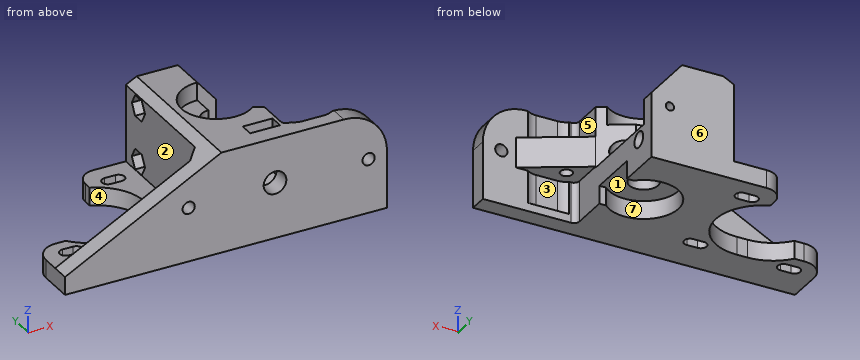
```python
from build123d import *

# Parameters (mm, degrees)
SKETCH1_R                = 4
BOSS_EXTRUDE1_DEPTH      = 28
SKETCH2_W                = 40.5
SKETCH2_H                = 38
CUT_EXTRUDE1_DEPTH       = 23
SKETCH3_R                = 9.65
CUT_EXTRUDE2_DEPTH       = 5
SKETCH8_R                = 1.15
CUT_EXTRUDE7_DEPTH       = 44
CHAMFER1_SIZE            = 23
CHAMFER1_SIZE2           = 43.5
SKETCH9_R                = 2.2
CUT_EXTRUDE8_DEPTH       = 90.5
CUT_EXTRUDE9_DEPTH       = 3
CUT_EXTRUDE9_DEPTH_BACK  = 4
CHAMFER2_SIZE            = 3
SKETCH16_W               = 26
SKETCH16_H               = 38
CUT_EXTRUDE12_DEPTH      = 29.0000001
CUT_EXTRUDE3_DEPTH       = 5
FILLET6_R                = 1.5
CUT_EXTRUDE13_DEPTH      = 17
SKETCH21_R               = 1.65
BOSS_EXTRUDE3_DEPTH      = 4.2
BOSS_EXTRUDE3_DEPTH_BACK = 4.2
SKETCH15_R               = 1.7
CUT_EXTRUDE11_DEPTH      = 44
CUT_EXTRUDE14_DEPTH      = 9
CHAMFER4_SIZE            = 8.5
CHAMFER4_SIZE2           = 10
FILLET1_R                = 5
FILLET2_R                = 6
FILLET4_R                = 12
CUT_EXTRUDE15_DEPTH      = 3.8
CUT_EXTRUDE18_REACH      = 45
SKETCH26_R               = 3.15


with BuildPart() as part:
    # Sketch1 → Boss-Extrude1 (new body)
    with BuildSketch(Plane.XY):
        with BuildLine():
            Line((-55, -23.6), (34.5, -23.6))
            Line((34.5, -23.6), (34.5, 19.4))
            Line((34.5, 19.4), (-28.5, 19.4))
            Line((-28.5, 19.4), (-28.5, 12.180409823))
            ThreePointArc((-28.5, 12.180409823), (-20.217668105, -2.285689125), (-33, -12.985083113))
            Line((-33, -12.985083113), (-36, -12.985083113))
            ThreePointArc((-36, -12.985083113), (-41.689100041, -11.672468641), (-46.228019527, -8))
            Line((-46.228019527, -8), (-55, -8))
            Line((-55, -8), (-55, -23.6))
        make_face()
        Circle(SKETCH1_R, mode=Mode.SUBTRACT)
        with BuildLine():
            Line((-23, 11.35), (-20, 11.35))
            ThreePointArc((-20, 11.35), (-18.35, 13), (-20, 14.65))
            Line((-20, 14.65), (-23, 14.65))
            ThreePointArc((-23, 14.65), (-24.65, 13), (-23, 11.35))
        make_face(mode=Mode.SUBTRACT)
        with BuildLine():
            Line((-23, -14.65), (-20, -14.65))
            ThreePointArc((-20, -14.65), (-18.35, -13), (-20, -11.35))
            Line((-20, -11.35), (-23, -11.35))
            ThreePointArc((-23, -11.35), (-24.65, -13), (-23, -14.65))
        make_face(mode=Mode.SUBTRACT)
        with BuildLine():
            Line((-46, -11.35), (-49, -11.35))
            ThreePointArc((-49, -11.35), (-50.65, -13), (-49, -14.65))
            Line((-49, -14.65), (-46, -14.65))
            ThreePointArc((-46, -14.65), (-44.35, -13), (-46, -11.35))
        make_face(mode=Mode.SUBTRACT)
    extrude(amount=BOSS_EXTRUDE1_DEPTH)

    # Sketch2 → Cut-Extrude1 (cut)
    with BuildSketch(Plane.XY.offset(28)):
        with Locations((-34.75, 0.4)):
            Rectangle(SKETCH2_W, SKETCH2_H)
    extrude(amount=-CUT_EXTRUDE1_DEPTH, mode=Mode.SUBTRACT)

    # Sketch3 → Cut-Extrude2 (cut)
    with BuildSketch(Plane.XY.offset(28)):
        Circle(SKETCH3_R)
    extrude(amount=-CUT_EXTRUDE2_DEPTH, mode=Mode.SUBTRACT)

    # Sketch8 → Cut-Extrude7 (cut, through all)
    with BuildSketch(Plane.XZ.offset(23.6)):
        with Locations((3.375, 15.5)):
            Circle(SKETCH8_R)
    extrude(amount=-CUT_EXTRUDE7_DEPTH, mode=Mode.SUBTRACT)

    # Chamfer1
    chamfer1_edges = [part.edges().sort_by_distance(p)[0] for p in [
        (-55, -21.1, 28),
    ]]
    chamfer1_side = [part.faces().sort_by_distance(p)[0] for p in [
        (-55, -18.958031088, 10.841968912),
    ]]
    chamfer(chamfer1_edges, length=CHAMFER1_SIZE, length2=CHAMFER1_SIZE2, reference=chamfer1_side[0])

    # Sketch9 → Cut-Extrude8 (cut, through all)
    with BuildSketch(Plane(origin=(34.5, 0, 0), x_dir=(0, 0, -1), z_dir=(1, 0, 0))):
        with Locations((-8, 13)):
            Circle(SKETCH9_R)
        with Locations((-23, 13)):
            Circle(SKETCH9_R)
    extrude(amount=-CUT_EXTRUDE8_DEPTH, mode=Mode.SUBTRACT)

    # Sketch10 → Cut-Extrude9 (cut, two sides)
    with BuildSketch(Plane.ZY.offset(14.5)) as cut_extrude9_sk:
        Polygon((5.1, 14.674315781), (5.1, 11.325684219), (8, 9.651368439), (10.9, 11.325684219), (10.9, 14.674315781), (8, 16.348631561), align=None)
        Polygon((25.9, 11.325684219), (25.9, 14.674315781), (23, 16.348631561), (20.1, 14.674315781), (20.1, 11.325684219), (23, 9.651368439), align=None)
    extrude(amount=CUT_EXTRUDE9_DEPTH, mode=Mode.SUBTRACT)
    extrude(cut_extrude9_sk.sketch, amount=-CUT_EXTRUDE9_DEPTH_BACK, mode=Mode.SUBTRACT)

    # Chamfer2
    chamfer2_edges = [part.edges().sort_by_distance(p)[0] for p in [
        (-14.5, -18.6, 15.706896552),
    ]]
    chamfer(chamfer2_edges, length=CHAMFER2_SIZE)

    # Sketch16 → Cut-Extrude12 (cut, through all)
    with BuildSketch(Plane.XY.offset(28)):
        with Locations((21.5, 0.4)):
            Rectangle(SKETCH16_W, SKETCH16_H)
    extrude(amount=-CUT_EXTRUDE12_DEPTH, mode=Mode.SUBTRACT)

    # Sketch4 → Cut-Extrude3 (cut)
    with BuildSketch(Plane(origin=(0, 0, 0), x_dir=(-1, 0, 0), z_dir=(0, 0, -1))):
        with BuildLine():
            Line((-36.31147183, -7), (-6.642476948, -7))
            ThreePointArc((-6.642476948, -7), (9.65, 0), (-6.642476948, 7))
            Line((-6.642476948, 7), (-36.31147183, 7))
            Line((-36.31147183, 7), (-36.31147183, -7))
        make_face()
    extrude(amount=-CUT_EXTRUDE3_DEPTH, mode=Mode.SUBTRACT)

    # Fillet6
    fillet6_edges = [part.edges().sort_by_distance(p)[0] for p in [
        (8.5, -18.6, 14),
    ]]
    fillet(fillet6_edges, radius=FILLET6_R)

    # Sketch17 → Cut-Extrude13 (cut)
    with BuildSketch(Plane.XY.offset(28)):
        with BuildLine():
            Line((0, 4), (0, 15.733500455))
            Line((0, 15.733500455), (8.5, 15.733500455))
            Line((8.5, 15.733500455), (8.5, -8.907477288))
            Line((8.5, -8.907477288), (0, -4))
            ThreePointArc((0, -4), (4, 0), (0, 4))
        make_face()
    extrude(amount=-CUT_EXTRUDE13_DEPTH, mode=Mode.SUBTRACT)

    # Sketch20 → Cut-Revolve1 (revolve, cut)
    with BuildSketch(Plane.XY.offset(15.5)):
        Polygon((3.375, -11.8), (7.375, -3.8), (3.375, -3.8), align=None)
    revolve(axis=Axis((3.375, -3.8, 15.5), (0, -1, 0)), mode=Mode.SUBTRACT)

    # Sketch21 → Boss-Extrude3 (add, two sides)
    with BuildSketch(Plane.XY.offset(15.5)) as boss_extrude3_sk:
        Polygon((7.25, -8.185789452), (7.25, -18.6), (25.287941791, -18.6), align=None)
        with Locations((13.25, -15)):
            Circle(SKETCH21_R, mode=Mode.SUBTRACT)
    extrude(amount=BOSS_EXTRUDE3_DEPTH)
    extrude(boss_extrude3_sk.sketch, amount=-BOSS_EXTRUDE3_DEPTH_BACK)

    # Sketch15 → Cut-Extrude11 (cut, through all)
    with BuildSketch(Plane.XZ.offset(23.6)):
        with Locations((-20.625, 15)):
            Circle(SKETCH15_R)
        with Locations((29.375, 15)):
            Circle(SKETCH15_R)
    extrude(amount=-CUT_EXTRUDE11_DEPTH, mode=Mode.SUBTRACT)

    # Sketch22 → Cut-Extrude14 (cut)
    with BuildSketch(Plane.XY.offset(19.7)):
        with BuildLine():
            Line((13.25, -19.5), (19.25, -19.5))
            ThreePointArc((19.25, -19.5), (23.75, -15), (19.25, -10.5))
            Line((19.25, -10.5), (13.25, -10.5))
            ThreePointArc((13.25, -10.5), (8.75, -15), (13.25, -19.5))
        make_face()
    cut_extrude14 = extrude(amount=CUT_EXTRUDE14_DEPTH, mode=Mode.SUBTRACT)

    # Mirror1: Cut-Extrude14 across plane
    add(cut_extrude14.mirror(Plane.XY.offset(15.5)), mode=Mode.SUBTRACT)

    # Chamfer4
    chamfer4_edges = [part.edges().sort_by_distance(p)[0] for p in [
        (8.5, 17.566750228, 28),
    ]]
    chamfer4_side = [part.faces().sort_by_distance(p)[0] for p in [
        (7.87031754, -13.003738644, 28),
    ]]
    chamfer(chamfer4_edges, length=CHAMFER4_SIZE, length2=CHAMFER4_SIZE2, reference=chamfer4_side[0])

    # Fillet1
    fillet1_edges = [part.edges().sort_by_distance(p)[0] for p in [
        (-28.5, 19.4, 2.5),
    ]]
    fillet(fillet1_edges, radius=FILLET1_R)

    # Fillet2
    fillet2_edges = [part.edges().sort_by_distance(p)[0] for p in [
        (-55, -8, 2.5),
    ]]
    fillet(fillet2_edges, radius=FILLET2_R)

    # Fillet4
    fillet4_edges = [part.edges().sort_by_distance(p)[0] for p in [
        (34.5, -21.1, 28),
    ]]
    fillet(fillet4_edges, radius=FILLET4_R)

    # Sketch23 → Cut-Extrude15 (cut)
    with BuildSketch(Plane.XZ.offset(18.6)):
        Polygon((-0.775, 28.722034997), (7.525, 28.722034997), (7.525, 13.103996383), (3.375, 10.707992766), (-0.775, 13.103996383), align=None)
    extrude(amount=-CUT_EXTRUDE15_DEPTH, mode=Mode.SUBTRACT)

    # Sketch26 → Cut-Extrude18 (cut, up to next)
    with BuildSketch(Plane.XZ.offset(23.6), mode=Mode.PRIVATE) as cut_extrude18_sk1:
        with Locations((3.375, 15.5)):
            Circle(SKETCH26_R)
    cut_extrude18_tool1 = extrude(cut_extrude18_sk1.sketch, amount=-CUT_EXTRUDE18_REACH, mode=Mode.PRIVATE) & part.part
    add(cut_extrude18_tool1.solids().sort_by_distance((3.375, -23.6, 15.5))[0], mode=Mode.SUBTRACT)


solid = part.part
```
Design review of the part built by this model. Coordinates are the model's own, in mm. Face numbers are marked on the shaded views. A direction names the side the tool comes from. Round coordinates to 2 decimals unless told otherwise and drop trailing zeros. Write each loop counter-clockwise with the first axis right and the second up, starting at its lowest first coordinate (ties: lowest second). Pieces come first, ordered by that corner, then holes. Notation, with made-up numbers: (-0.5, 57.5) -> (27.5, 57.5) arc R25 ccw to (27.5, 73.5) -> close; hole circle Ø2 at (-15, 61.25). An arc over 180 degrees is marked (long way). Write item = value, one per line. Start each with the question number.
1) Clearance check with flat-ended pins moving along their axes: pin 1 (1.5 mm diameter, centred on y = 11, z = 24.5, fed in from +X); pin 2 (8.5 mm diameter, centred on x = 17.5, y = -14.5, fed in from +Z); pin 3 (2 mm diameter, centred on y = -19, z = 21, fed in from +X); pin 4 (1.4 mm diameter, centred on x = 3.375, z = 15.5, fed in from -Y). State where each tip first meets the part, or that it passes through.
2) Take a section at A-A, the plane y = 0. State the section outline as (x, z) points.
3) Wall thickness on probe 1 along Y at (x, z) = (-0.25, 8); probe 2 along Y at (x, z) = (0, 1.8); probe 3 along X at (y, z) = (-21.5, 13.75): over which ranges is each line inside the solid? List them lowest first. Write a range as from..to.
4) Take a section at B-B, the plane x = 20.5. State the section outline as (y, z) points.
5) Mouldability with a two-part tool opening along X and no side actions: class the marked faces 4, 5, 6 and 7 as +X half, -X half, draft (parallel to the pull), parting line (faces both ways), or undercut.
6) Tool access review of the marked faces 1, 2 and 3: name each direction out of +Z, -Z, +X, -X, +Y, -Y from which nothing blocks a thin tool from reaching the whole face with its end or side.
Results list:
q1.pin_1 = 0
q1.pin_2 = 19.7
q1.pin_3 = 33.81
q1.pin_4 = through
q2.outline = (-20.01, 0) -> (-9.65, 0) -> (-9.65, 5) -> (-4, 5) -> (-4, 23) -> (-9.65, 23) -> (-9.65, 28) -> (-11.5, 28) -> (-14.5, 26.41) -> (-14.5, 5) -> (-20.01, 5) -> close; (4, 5) -> (8.5, 5) -> (8.5, 11) -> (4, 11) -> close
q3.probe_1 = -23.6..-3.99, 3.99..10.8, 15.2..19.4
q3.probe_2 = -23.6..-9.65, 9.65..19.4
q3.probe_3 = -38.45..-21.78, -19.47..0.76, 5.99..28.22, 30.53..34.5
q4.outline = (-23.6, 0) -> (-18.6, 0) -> (-18.6, 2.3) -> (-19.32, 2.3) -> (-19.32, 11.3) -> (-15.84, 11.3) -> (-15.84, 19.7) -> (-19.32, 19.7) -> (-19.32, 28) -> (-23.6, 28) -> close
q5.face_4 = undercut
q5.face_5 = +X half
q5.face_6 = draft
q5.face_7 = undercut
q6.face_1 = -Z
q6.face_2 = +Z, -X, +Y
q6.face_3 = +Y
